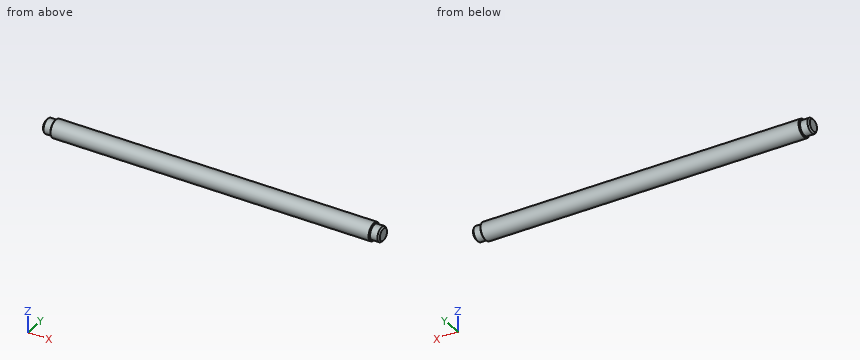
from build123d import *

# Parameters (mm, degrees)
CHAMFER1_SIZE = 0.2
CHAMFER2_SIZE = 0.2
CHAMFER3_SIZE = 0.5
CHAMFER4_SIZE = 0.5


with BuildPart() as part:
    # Sketch1 → Revolve1 (revolve)
    with BuildSketch(Plane.XY, mode=Mode.PRIVATE) as revolve1_sk:
        Polygon((0, 0), (115, 0), (115, 2.5), (112, 2.5), (112, 3), (3, 3), (3, 2.5), (0, 2.5), align=None)
    revolve(revolve1_sk.sketch.rotate(Axis((0, 0, 0), (1, 0, 0)), 90), axis=Axis((0, 0, 0), (1, 0, 0)))

    # Chamfer1
    chamfer1_edges = [part.edges().sort_by_distance(p)[0] for p in [
        (112, 0, -3),
    ]]
    chamfer(chamfer1_edges, length=CHAMFER1_SIZE)

    # Chamfer2
    chamfer2_edges = [part.edges().sort_by_distance(p)[0] for p in [
        (3, 0, -3),
    ]]
    chamfer(chamfer2_edges, length=CHAMFER2_SIZE)

    # Chamfer3
    chamfer3_edges = [part.edges().sort_by_distance(p)[0] for p in [
        (0, 0, -2.5),
    ]]
    chamfer(chamfer3_edges, length=CHAMFER3_SIZE)

    # Chamfer4
    chamfer4_edges = [part.edges().sort_by_distance(p)[0] for p in [
        (115, 0, -2.5),
    ]]
    chamfer(chamfer4_edges, length=CHAMFER4_SIZE)


solid = part.part
Geometry check sheet. Reference: the model listing, model coordinates, mm. Coordinates: 2 decimals unless noted, no trailing zeros. Order: outer loops, then holes, each group sorted by start corner. A loop starts at its lowest first (then second) coordinate and runs counter-clockwise, first axis right, second up. Notation, with made-up numbers: (7, 14) - (64, 14) arc R20 ccw to (64, 26) - close; hole circle Ø3 at (-20, -2). An arc over 180 degrees is marked (long way). One line per item, written item: value.
(1) Thickness scan on probe 1 along Z at (x, y) = (9, 2.25); probe 2 along Y at (x, z) = (38, 0.1); probe 3 along X at (y, z) = (-0.75, -2.5). Record the ranges inside material, lowest first. Write a range as from..to.
Data:
probe 1: z = -1.98..1.98
probe 2: y = -3..3
probe 3: x = 3..112
(2) Depth check by flat-ended pin: pin 1 Ø1 at (y, z) = (-2, 2.5) entering from +X. Enter the tip coordinate at first touch or a pass-through.
Data:
pin 1: stops at x = 112
(3) Sectioned sample at A-A (x = 102.5). Enter the section's corners in (y, z), and give its area (3 significant figures).
Data:
outline: circle Ø6 at (0, 0)
area: 28.3 mm^2
